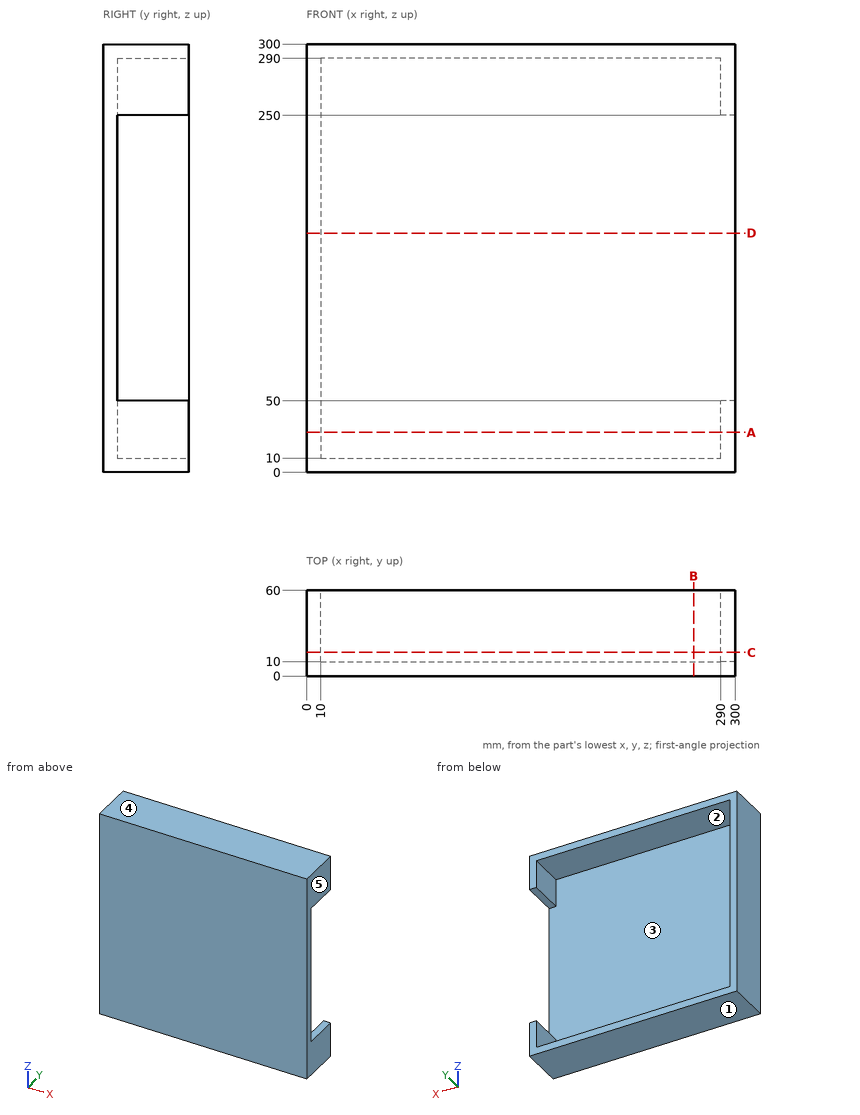
Could you check a few things on this drawing? It's one solid part, dimensions in mm from its lowest x, y, z. A direction names the side the tool comes from. Give positions to 0.01 mm unless a question says otherwise; leave off trailing zeros. Loops run counter-clockwise (first coordinate to the right, second up) from the corner with the lowest first, then second, coordinate; pieces in that order, holes last. Notation, with made-up numbers: M -3.5,43.5 L 24.5,43.5 A24 cw 24.5,65.5 Z; hole C 5.5,79 d11. An arc over 180 degrees is marked long. Return JSON: item names as keys, results as strings.
Item 1: I'm going to push a flat-ended pin straight in: pin 1 Ø10 at (x, z) = (240, 230) entering from +Y. Where does the tip first touch, or does it pass through?
A:
{"pin 1": "stops at y = 10"}
Item 2: Imagine slicing it at D-D on z = 167.5. List the corners of the cut face in (x, y) for me.
A:
{"outline": "M 0,0 L 300,0 L 300,10 L 10,10 L 10,60 L 0,60 Z"}
Item 3: Imagine slicing it at A-A on z = 28. List the corners of the cut face in (x, y) for me.
A:
{"outline": "M 0,0 L 300,0 L 300,60 L 290,60 L 290,10 L 10,10 L 10,60 L 0,60 Z"}
Item 4: Imagine slicing it at C-C on y = 16.5. List the corners of the cut face in (x, z) for me.
A:
{"outline": "M 0,0 L 300,0 L 300,50 L 290,50 L 290,10 L 10,10 L 10,290 L 290,290 L 290,250 L 300,250 L 300,300 L 0,300 Z"}
Item 5: On a 3-axis mill with a long thin cutter (end or side, diameter ignored), from which of +Z, -Z, +X, -X, +Y, -Y can I reach the whole of each face in a straight line? I mean the marked faces 1 and 2. Say none if no direction works.
A:
{"face 1": "-Z, +X, -X, +Y, -Y", "face 2": "+Y"}
Item 6: Please list where these lines run through material, in increasing order: line 1 (Z direction, x = 264, y = 31.5); line 2 (Y direction, x = 25, z = 32).
A:
{"line 1": "z = 0 to 10, 290 to 300", "line 2": "y = 0 to 10"}
Item 7: Imagine slicing it at B-B on x = 271. List the corners of the cut face in (y, z) for me.
A:
{"outline": "M 0,0 L 60,0 L 60,10 L 10,10 L 10,290 L 60,290 L 60,300 L 0,300 Z"}
Item 8: Thinking about a two-plate mould opening in X: for the marked faces 3, 4 and 5, which applies, released by +X, released by -X, zero draft, split by the parting line, or undercut?
A:
{"face 3": "undercut", "face 4": "zero draft", "face 5": "released by +X"}
